Source: three-view drawing plus pictorial views. Frame: mm from the lowest corner of the part. Coordinates: 2 decimals unless noted, no trailing zeros. Order: outer loops, then holes, each group sorted by start corner. A loop starts at its lowest first (then second) coordinate and runs counter-clockwise, first axis right, second up. Notation, with made-up numbers: (7.5, 35.5) - (55.5, 35.5) arc R35 ccw to (55.5, 71.5) - close; hole circle Ø9 at (11, 32.5). An arc over 180 degrees is marked (long way). One line per question, with ' | ' between items.
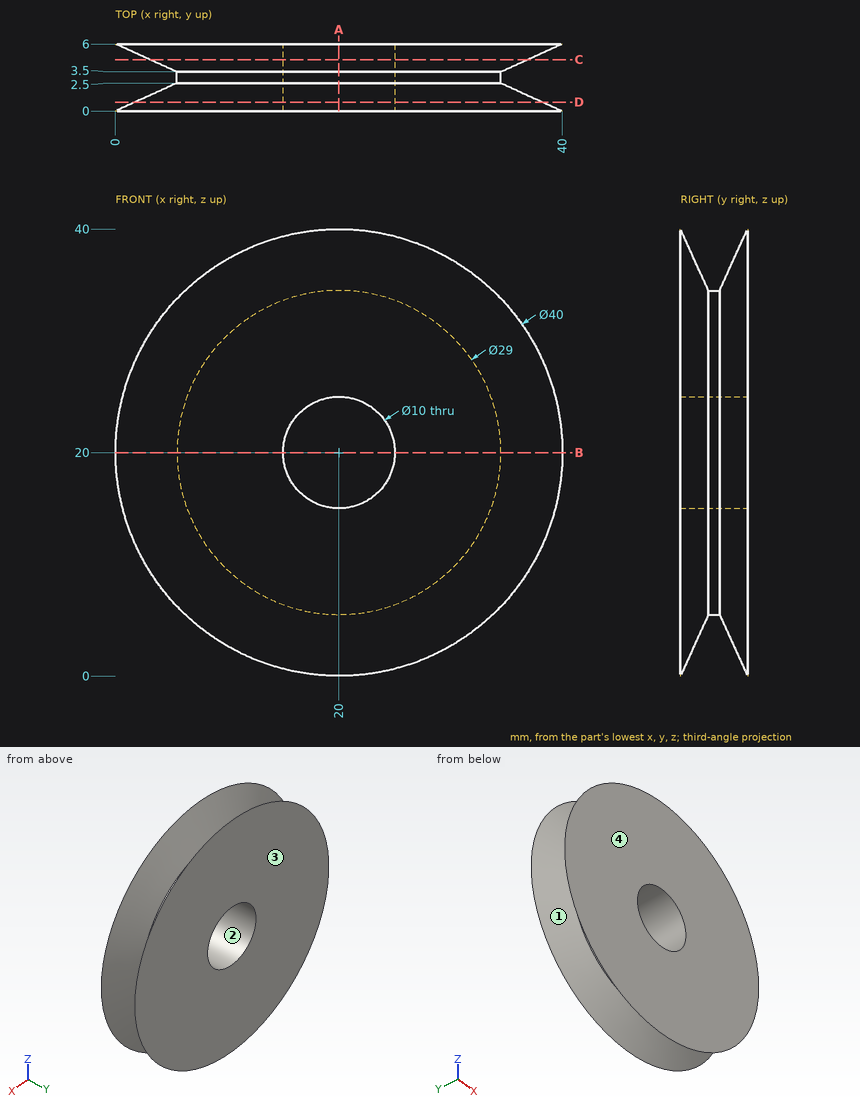
Item 1: Section C-C on y = 4.6. Return the cut outline in (x, z), and give its area (3 significant figures).
Data:
outline: circle Ø33.84 at (20, 20); hole circle Ø10 at (20, 20) | area: 821 mm^2
Item 2: Section B-B on z = 20. Return the cut outline in (x, y), and give its area (4 significant figures).
Data:
outline: (0, 0) - (15, 0) - (15, 6) - (0, 6) - (5.5, 3.5) - (5.5, 2.5) - close; (25, 0) - (40, 0) - (34.5, 2.5) - (34.5, 3.5) - (40, 6) - (25, 6) - close | area: 141.5 mm^2
Item 3: Contact query for flat-ended pins moving along their axis: P1, Ø10, axis at x = 11.5, z = 9, coming from the -Y side; P2, Ø1, axis at y = 3, z = 7.5, coming from the -X side; P3, Ø1.5, axis at x = 21.5, y = 4, coming from the +Z side. Output: stop coordinate, or through.
Data:
P1: y = 0 | P2: x = 11.86 | P3: z = 37.19
Item 4: Section D-D on y = 0.8. Return the cut outline in (x, z), and give its area (3 significant figures).
Data:
outline: circle Ø36.48 at (20, 20); hole circle Ø10 at (20, 20) | area: 967 mm^2
Item 5: Section A-A on x = 20. Return the cut outline in (y, z).
Data:
outline: (0, 0) - (2.5, 5.5) - (3.5, 5.5) - (6, 0) - (6, 15) - (0, 15) - close; (0, 25) - (6, 25) - (6, 40) - (3.5, 34.5) - (2.5, 34.5) - (0, 40) - close
Item 6: Draft query along Y for the marked faces 1, 2, 3 and 4. Return one class per face: released by +Y, released by -Y, zero draft, split by the parting line, or undercut.
Data:
face 1: undercut | face 2: zero draft | face 3: released by +Y | face 4: released by -Y
Item 7: Ray query, line 1 (Z direction, x = 20, y = 2.65); line 2 (Z direction, x = 20, y = 3.95). Return the intervals inside material, ascending.
Data:
line 1: 5.5 to 15, 25 to 34.5 | line 2: 4.51 to 15, 25 to 35.49
